```python
from build123d import *

# Parameters (mm, degrees)
SKETCH_W             = 132.4
SKETCH_H             = 118.2
PAD_DEPTH            = 4
PAD_DEPTH_BACK       = 10
SKETCH001_W          = 124.4
SKETCH001_H          = 114.2
POCKET_DEPTH         = 10.001
SKETCH002_W          = 116.4
SKETCH002_H          = 110.2
POCKET001_DEPTH      = 5
FILLET_R             = 6
FILLET001_R          = 10
FILLET002_R          = 2
POCKET002_DEPTH      = 10.001
POCKET002_DEPTH_BACK = 4.001
PAD001_DEPTH         = 10
SKETCH005_W          = 1
SKETCH005_H          = 8
POCKET003_DEPTH      = 10.001
POCKET003_DEPTH_BACK = 4.001
SKETCH006_R          = 1.65
POCKET004_DEPTH      = 66.201
POCKET004_DEPTH_BACK = 66.201
POCKET005_DEPTH      = 64.5
SKETCH008_R          = 1.65
POCKET006_DEPTH      = 59.101
POCKET006_DEPTH_BACK = 59.101
POCKET007_DEPTH      = 57.4
SKETCH010_W          = 124.4
SKETCH010_H          = 13
SKETCH010_H_2        = 26
SKETCH010_W_2        = 26
SKETCH010_H_3        = 4
POCKET008_DEPTH      = 4.001
FILLET003_R          = 3


with BuildPart() as part:
    # Sketch → Pad (new body, two sides)
    with BuildSketch(Plane.XY) as pad_sk:
        Rectangle(SKETCH_W, SKETCH_H)
    extrude(amount=PAD_DEPTH)
    extrude(pad_sk.sketch, amount=-PAD_DEPTH_BACK)

    # Sketch001 → Pocket (cut, through all)
    with BuildSketch(Plane.XY):
        with Locations((0, -2)):
            Rectangle(SKETCH001_W, SKETCH001_H)
    extrude(amount=-POCKET_DEPTH, mode=Mode.SUBTRACT)

    # Sketch002 → Pocket001 (cut)
    with BuildSketch(Plane.XY):
        with Locations((0, -4)):
            Rectangle(SKETCH002_W, SKETCH002_H)
    extrude(amount=POCKET001_DEPTH, mode=Mode.SUBTRACT)

    # Fillet
    fillet_edges = [part.edges().sort_by_distance(p)[0] for p in [
        (-62.2, 55.1, -5),
        (62.2, 55.1, -5),
    ]]
    fillet(fillet_edges, radius=FILLET_R)

    # Fillet001
    fillet001_edges = [part.edges().sort_by_distance(p)[0] for p in [
        (-66.2, 59.1, -3),
        (66.2, 59.1, -3),
    ]]
    fillet(fillet001_edges, radius=FILLET001_R)

    # Fillet002
    fillet002_edges = [part.edges().sort_by_distance(p)[0] for p in [
        (-58.2, 51.1, 2),
        (58.2, 51.1, 2),
    ]]
    fillet(fillet002_edges, radius=FILLET002_R)

    # Sketch003 → Pocket002 (cut, two sides)
    with BuildSketch(Plane.XY) as pocket002_sk:
        with BuildLine():
            Line((-65.2, 39.1), (-65.2, 49.1))
            ThreePointArc((-56.2, 58.1), (-62.563961, 55.463961), (-65.2, 49.1))
            Line((-46.2, 58.1), (-56.2, 58.1))
            Line((-46.2, 58.1), (-46.2, 59.1))
            Line((-46.2, 59.1), (-56.2, 59.1))
            ThreePointArc((-56.2, 59.1), (-63.271068, 56.171068), (-66.2, 49.1))
            Line((-66.2, 39.1), (-66.2, 49.1))
            Line((-65.2, 39.1), (-66.2, 39.1))
        make_face()
        with BuildLine():
            Line((65.2, 39.1), (65.2, 49.1))
            ThreePointArc((65.2, 49.1), (62.563961, 55.463961), (56.2, 58.1))
            Line((46.2, 58.1), (56.2, 58.1))
            Line((46.2, 58.1), (46.2, 59.1))
            Line((46.2, 59.1), (56.2, 59.1))
            ThreePointArc((66.2, 49.1), (63.271068, 56.171068), (56.2, 59.1))
            Line((66.2, 39.1), (66.2, 49.1))
            Line((65.2, 39.1), (66.2, 39.1))
        make_face()
    extrude(amount=-POCKET002_DEPTH, mode=Mode.SUBTRACT)
    extrude(pocket002_sk.sketch, amount=POCKET002_DEPTH_BACK, mode=Mode.SUBTRACT)

    # Sketch004 → Pad001 (join)
    with BuildSketch(Plane.XY):
        Polygon((-62.2, 24.7), (-62.2, 26.1), (-60.55, 27), (-60.55, 23.8), align=None)
        Polygon((-62.2, 5.7), (-60.55, 4.8), (-60.55, 8), (-62.2, 7.1), align=None)
        Polygon((-62.2, -50.3), (-60.55, -51.2), (-60.55, -48), (-62.2, -48.9), align=None)
        Polygon((62.2, 24.7), (62.2, 26.1), (60.55, 27), (60.55, 23.8), align=None)
        Polygon((62.2, 5.7), (60.55, 4.8), (60.55, 8), (62.2, 7.1), align=None)
        Polygon((62.2, -50.3), (60.55, -51.2), (60.55, -48), (62.2, -48.9), align=None)
    extrude(amount=-PAD001_DEPTH)

    # Sketch005 → Pocket003 (cut, two sides)
    with BuildSketch(Plane.XY) as pocket003_sk:
        with Locations((-65.7, -55.1)):
            Rectangle(SKETCH005_W, SKETCH005_H)
        with Locations((65.7, -55.1)):
            Rectangle(SKETCH005_W, SKETCH005_H)
    extrude(amount=-POCKET003_DEPTH, mode=Mode.SUBTRACT)
    extrude(pocket003_sk.sketch, amount=POCKET003_DEPTH_BACK, mode=Mode.SUBTRACT)

    # Sketch006 → Pocket004 (cut, two sides)
    with BuildSketch(Plane.YZ) as pocket004_sk:
        with Locations((-55.1, -4)):
            Circle(SKETCH006_R)
        with Locations((44.1, -4)):
            Circle(SKETCH006_R)
    extrude(amount=-POCKET004_DEPTH, mode=Mode.SUBTRACT)
    extrude(pocket004_sk.sketch, amount=POCKET004_DEPTH_BACK, mode=Mode.SUBTRACT)

    # Sketch007 → Pocket005 (cut, symmetric)
    with BuildSketch(Plane.YZ):
        Polygon((-57.975, -5.659882), (-55.1, -7.319764), (-52.225, -5.659882), (-52.225, -2.340118), (-55.1, -0.680236), (-57.975, -2.340118), align=None)
        Polygon((44.1, -7.319764), (46.975, -5.659882), (46.975, -2.340118), (44.1, -0.680236), (41.225, -2.340118), (41.225, -5.659882), align=None)
    extrude(amount=POCKET005_DEPTH, both=True, mode=Mode.SUBTRACT)

    # Sketch008 → Pocket006 (cut, two sides)
    with BuildSketch(Plane.XZ) as pocket006_sk:
        with Locations((-51.2, -4)):
            Circle(SKETCH008_R)
        with Locations((51.2, -4)):
            Circle(SKETCH008_R)
    extrude(amount=-POCKET006_DEPTH, mode=Mode.SUBTRACT)
    extrude(pocket006_sk.sketch, amount=POCKET006_DEPTH_BACK, mode=Mode.SUBTRACT)

    # Sketch009 → Pocket007 (cut)
    with BuildSketch(Plane.XZ):
        Polygon((-51.2, -7.319764), (-48.325, -5.659882), (-48.325, -2.340118), (-51.2, -0.680236), (-54.075, -2.340118), (-54.075, -5.659882), align=None)
        Polygon((51.2, -7.319764), (54.075, -5.659882), (54.075, -2.340118), (51.2, -0.680236), (48.325, -2.340118), (48.325, -5.659882), align=None)
    extrude(amount=-POCKET007_DEPTH, mode=Mode.SUBTRACT)

    # Sketch010 → Pocket008 (cut, through all)
    with BuildSketch(Plane.XY):
        with Locations((0, -52.6)):
            Rectangle(SKETCH010_W, SKETCH010_H)
        with Locations((0, 15.9)):
            Rectangle(SKETCH010_W, SKETCH010_H_2)
        with Locations((-35, 53.1)):
            Rectangle(SKETCH010_W_2, SKETCH010_H_3)
        with Locations((35, 53.1)):
            Rectangle(SKETCH010_W_2, SKETCH010_H_3)
    extrude(amount=POCKET008_DEPTH, mode=Mode.SUBTRACT)

    # Fillet003
    fillet003_edges = [part.edges().sort_by_distance(p)[0] for p in [
        (-58.2, -46.1, 2),
        (-58.2, 2.9, 2),
        (-58.2, 28.9, 2),
        (-48, 51.1, 2),
        (-22, 51.1, 2),
        (22, 51.1, 2),
        (48, 51.1, 2),
        (58.2, 28.9, 2),
        (58.2, 2.9, 2),
        (58.2, -46.1, 2),
    ]]
    fillet(fillet003_edges, radius=FILLET003_R)


solid = part.part
```
Work out the finished part from the listing and answer in its coordinate system (mm). A direction names the side the tool comes from. Round coordinates to 2 decimals unless told otherwise and drop trailing zeros. Order: outer loops, then holes, each group sorted by start corner. A loop starts at its lowest first (then second) coordinate and runs counter-clockwise, first axis right, second up.
Q1. Find the intervals of material crossed by line 1 along Z through (x, y) = (51.2, 57.75); line 2 along X through (y, z) = (-42.5, 1); line 3 along X through (y, z) = (-21.5, -8.25), in increasing order.
Solution:
line 1: z = -10 to -5.65, -2.35 to 4
line 2: x = -66.2 to -58.2, 58.2 to 66.2
line 3: x = -66.2 to -62.2, 62.2 to 66.2
Q2. A cutting plane is placed at A-A, the plane y = 37.5. Determine the outline of the cut face in (x, z).
Solution:
outline: (-66.2, -10) - (-62.2, -10) - (-62.2, 0) - (-58.2, 0) - (-58.2, 4) - (-66.2, 4) - close; (58.2, 0) - (62.2, 0) - (62.2, -10) - (66.2, -10) - (66.2, 4) - (58.2, 4) - close
Q3. A tool of negligible diameter and unlimited length cuts with its end or side. For faces 1 (the cylindrical face through (-60.489, 53.296, -5.07)), 2 (the cylindrical face through (-59.1, 29.76, 1.97)), 3 (the flat face through (51, 58.1, -2)), 4 (the flat face through (-58.2, -22, 2)), 5 (the flat face through (64, -59.1, -3)), from which of +Z, -Z, +X, -X, +Y, -Y can it reach the whole face along a straight path? Write none if from no direction.
Solution:
face 1: -Z
face 2: +Z, -Z
face 3: +Z, -Z, +X, +Y
face 4: +Z, -Z, -Y
face 5: +Z, -Z, +X, -X, -Y
Q4. A cutting plane is placed at B-B, the plane z = -4. Count the separate pieces of the cut face and the enclosed holes in it, then the cut area to 3 significant figures.
Solution:
separate pieces: 7
enclosed holes: 0
area: 1,260 mm2
Q5. Given pin 1 Ø1.8 at (y, z) = (56, -4.5) entering from +X; pin 2 Ø4 at (x, z) = (-49, -3) entering from -Y; pin 3 Ø4 at (x, z) = (-16.5, 2) entering from -Y, each flat-ended and moving along its own axis, determine where each tip first touches the part or whether it passes through.
Solution:
pin 1: stops at x = 62.91
pin 2: stops at y = 55.1
pin 3: stops at y = 51.1
Q6. The mould has two halves that part along Z. Classify faces 6 (the cylindrical face through (21.1, 51.96, 2.03)), 7 (the flat face through (59, 44, 0)), 8 (the flat face through (-64.5, 42.8, -5.4)), 9 (the flat face through (64.5, -56.4, -5.4)): pulls with the +Z half, pulls with the -Z half, needs draft (parallel to the pull), parting line crosses it, or undercut.
Solution:
face 6: needs draft
face 7: pulls with the -Z half
face 8: undercut
face 9: undercut
